```python
from build123d import *

# Parameters (mm, degrees)
SKETCH4_R                  = 3
BOSS_EXTRUDE1_DEPTH        = 21.59
CUT_EXTRUDE1_START         = -15.24
SKETCH8_R                  = 3.175
CUT_EXTRUDE1_DEPTH         = 5.08
F_10_32_TAPPED_HOLE1_D     = 4.0386
F_10_32_TAPPED_HOLE1_DEPTH = 13.8176
F_10_32_TAPPED_HOLE1_TIP   = 1.213317848


with BuildPart() as part:
    # Sketch4 → Boss-Extrude1 (new body)
    with BuildSketch(Plane(origin=(0, 0, 0), x_dir=(0, 0, -1), z_dir=(1, 0, 0))):
        with BuildLine():
            Line((3.667013126, -26.3254835), (2.816473307, -8.431236894))
            ThreePointArc((2.816473307, -8.431236894), (1.639602622, -6.396649217), (-0.700777066, -6.179406175))
            add(Edge.make_bspline(
                [(-0.700777066, -6.179406175), (-1.525102008, -6.512822326), (-2.494871997, -6.679047096), (-4.555429578, -6.54165034), (-5.644996058, -6.237076936), (-7.717261628, -5.106975392), (-8.698405735, -4.281093265), (-10.311829803, -2.164612563), (-10.942499326, -0.874358563), (-11.647480976, 2.006859472), (-11.720427957, 3.596803483), (-11.182779689, 6.826310345), (-10.571334953, 8.46432492), (-9.132019695, 10.73433891), (-8.566197708, 11.459621106), (-7.273120414, 12.810057002), (-6.545872807, 13.435152517), (-4.948692799, 14.549748502), (-4.078780417, 15.039192621), (-2.22269385, 15.85074605), (-1.236551533, 16.172803424), (0.818678144, 16.623204755), (1.887722789, 16.751503646), (4.069669804, 16.79483508), (5.182520117, 16.709831654), (7.408648574, 16.315055224), (8.521867273, 16.00525724), (10.70264063, 15.158359498), (11.770130786, 14.621247223), (13.812561896, 13.326727542), (14.787435905, 12.56932106), (16.598938448, 10.850935673), (17.435500393, 9.889971566), (18.927885533, 7.790674993), (19.583645356, 6.652371052), (20.677096627, 4.233429246), (21.114730733, 2.952832896), (21.741586229, 0.292117033), (21.930758945, -1.087949282), (22.038932986, -3.898444365), (21.957896657, -5.328810088), (21.513783431, -8.186144708), (21.150681858, -9.613043017), (20.141400668, -12.407098951), (19.49521083, -13.774181132), (17.930076055, -16.391877744), (17.011136269, -17.642414844), (14.922264044, -19.972214517), (13.752352434, -21.051401006), (11.194349378, -22.98792657), (9.80629411, -23.845193985), (6.855009859, -25.29377098), (5.291831431, -25.88501641), (3.667013126, -26.3254835)],
                knots=[0, 0, 0, 0, 0.0625, 0.0625, 0.125, 0.125, 0.1875, 0.1875, 0.25, 0.25, 0.3125, 0.3125, 0.375, 0.375, 0.40625, 0.40625, 0.4375, 0.4375, 0.46875, 0.46875, 0.5, 0.5, 0.53125, 0.53125, 0.5625, 0.5625, 0.59375, 0.59375, 0.625, 0.625, 0.65625, 0.65625, 0.6875, 0.6875, 0.71875, 0.71875, 0.75, 0.75, 0.78125, 0.78125, 0.8125, 0.8125, 0.84375, 0.84375, 0.875, 0.875, 0.90625, 0.90625, 0.9375, 0.9375, 0.96875, 0.96875, 1, 1, 1, 1], degree=3))
        make_face()
        Circle(SKETCH4_R, mode=Mode.SUBTRACT)
    extrude(amount=BOSS_EXTRUDE1_DEPTH)

    # Sketch8 → Cut-Extrude1 (cut)
    with BuildSketch(Plane(origin=(0, 0, 0), x_dir=(1, 0, 0), z_dir=(0, -0.99887229, -0.047477867)).offset(CUT_EXTRUDE1_START)):
        with Locations((16.565, 0)):
            Circle(SKETCH8_R)
    extrude(amount=-CUT_EXTRUDE1_DEPTH, mode=Mode.SUBTRACT)

    # 10-32 Tapped Hole1
    with Locations(Plane(origin=(0, 15.222813703, 0.72356269), x_dir=(1, 0, 0), z_dir=(0, 0.99887229, 0.047477867))):
        with Locations((16.565, 0)):
            Hole(F_10_32_TAPPED_HOLE1_D / 2, depth=F_10_32_TAPPED_HOLE1_DEPTH)
            with Locations((0, 0, -(F_10_32_TAPPED_HOLE1_DEPTH + F_10_32_TAPPED_HOLE1_TIP / 2))):  # 118° drill point
                Cone(0, F_10_32_TAPPED_HOLE1_D / 2, F_10_32_TAPPED_HOLE1_TIP, mode=Mode.SUBTRACT)


solid = part.part
```
Geometry: final body of the model. Coordinates: model frame, mm. Round coordinates to 2 decimals unless told otherwise and drop trailing zeros. Use CSV: the item, a comma, the result in double quotes. Start each with the question number.
1) First-contact query: pin 1 Ø2 at (x, y) = (15, 8.5) entering from +Z; pin 2 Ø8 at (y, z) = (4.5, -2.5) entering from -X; pin 3 Ø10 at (x, z) = (10.5, -6) entering from +Y; pin 4 Ø3.5 at (y, z) = (0, 0) entering from +X. Flat tips, straight axial feed; report the tip coordinate or a pass-through.
2) Draft query along Y for faces 1 (the face through (15.88, 15.9, -2.35)), 2 (the face through (0, 0, -5)), 3 (the face through (10.644, -6.415, -1.668)). Return one class per face: +Y half, -Y half, draft (parallel to the pull), parting line (faces both ways), or undercut.
3) Section A-A (z = 1.5). State how many separate pieces and enclosed holes the cut face has, and give its area (3 significant figures).
4) Material intervals for line 1 along Y through (x, z) = (10.5, 0); line 2 along Z through (x, y) = (11.5, 9.5); line 3 along Y through (x, z) = (2, -4), sorted ascending. Write a range as from..to.
Returned:
1,pin 1,"stops at z = 10.84"
1,pin 2,"stops at x = 0"
1,pin 3,"stops at y = 16.78"
1,pin 4,"passes through"
2,face 1,"undercut"
2,face 2,"draft"
2,face 3,"-Y half"
3,separate pieces,"3"
3,enclosed holes,"0"
3,area,"325 mm²"
4,line 1,"y = -6.01..-3, 3..16.44"
4,line 2,"z = -17.69..9.9"
4,line 3,"y = -26.23..16.76"
